from build123d import *

# Parameters (mm, degrees)
SKETCH1_W                        = 50.8
SKETCH1_H                        = 76.2
SKETCH1_R                        = 14.2875
BOSS_EXTRUDE1_DEPTH              = 8.89
F_10_CLEARANCE_HOLE1_D           = 5.1054
F_10_CLEARANCE_HOLE1_CSINK_D     = 6.3754
F_10_CLEARANCE_HOLE1_CSINK_ANGLE = 90


with BuildPart() as part:
    # Sketch1 → Boss-Extrude1 (new body)
    with BuildSketch(Plane.XY):
        with Locations((25.4, 38.1)):
            Rectangle(SKETCH1_W, SKETCH1_H)
        with Locations((25.4, 38.1)):
            Circle(SKETCH1_R, mode=Mode.SUBTRACT)
    extrude(amount=BOSS_EXTRUDE1_DEPTH)

    # #10 Clearance Hole1 (through all)
    with Locations(Plane.XY.offset(8.89)):
        with Locations((25.4, 66.675), (25.4, 9.525)):
            CounterSinkHole(F_10_CLEARANCE_HOLE1_D / 2, F_10_CLEARANCE_HOLE1_CSINK_D / 2, counter_sink_angle=F_10_CLEARANCE_HOLE1_CSINK_ANGLE)


solid = part.part
The model under review builds one solid part; all positions refer to its coordinate system, in mm. Give positions to 0.01 mm unless a question says otherwise; leave off trailing zeros. Order: outer loops, then holes, each group sorted by start corner. A loop starts at its lowest first (then second) coordinate and runs counter-clockwise, first axis right, second up. Notation, with made-up numbers: M 10.25,-4 L 68.25,-4 A24 cw 68.25,25 Z; hole C -5.5,52.5 d7. An arc over 180 degrees is marked long. Use one line per item in the form item = value. Start each with the question number.
Item 1: We need section A-A on x = 25.4. Give the boundary of the cut face in (y, z) (1 decimal).
Item 2: The part is to be moulded in two halves that separate along Y. For faces 1 (the flat face through (25, 76.2, 4)), 2 (the cylindrical face through (27.95, 9.64, 4.07)), 3 (the flat face through (50.8, 38, 4)), 4 (the cylindrical face through (14.06, 29.41, 4.38)), say which applies: pulls with the +Y half, pulls with the -Y half, needs draft (parallel to the pull), parting line crosses it, or undercut.
Item 3: We need section D-D on z = 7. Give the boundary of the cut face in (x, y) (1 decimal).
Item 4: We need section C-C on x = 35. Give the boundary of the cut face in (y, z), plus the area to 3 significant figures.
Item 5: To check wall thickness, follow line 1 along Y through (x, z) = (25.4, 5.5); line 2 along X through (y, z) = (66.5, 0.75); line 3 along Y through (x, z) = (34.5, 8.25). State the ranges of each line that lie inside material, in increasing order. Write a range as from..to.
Item 6: We need section B-B on y = 38.1. Give the boundary of the cut face in (x, z).
Completed:
q1.outline = M 0,0 L 7,0 L 7,8.3 L 6.3,8.9 L 0,8.9 Z; M 12.1,0 L 23.8,0 L 23.8,8.9 L 12.7,8.9 L 12.1,8.3 Z; M 52.4,0 L 64.1,0 L 64.1,8.3 L 63.5,8.9 L 52.4,8.9 Z; M 69.2,0 L 76.2,0 L 76.2,8.9 L 69.9,8.9 L 69.2,8.3 Z
q2.face_1 = pulls with the +Y half
q2.face_2 = undercut
q2.face_3 = needs draft
q2.face_4 = undercut
q3.outline = M 0,0 L 50.8,0 L 50.8,76.2 L 0,76.2 Z; hole C 25.4,38.1 d28.6; hole C 25.4,9.5 d5.1; hole C 25.4,66.7 d5.1
q4.outline = M 0,0 L 27.52,0 L 27.52,8.89 L 0,8.89 Z; M 48.68,0 L 76.2,0 L 76.2,8.89 L 48.68,8.89 Z
q4.area = 489 mm²
q5.line_1 = 0..6.97, 12.08..23.81, 52.39..64.12, 69.23..76.2
q5.line_2 = 0..22.85, 27.95..50.8
q5.line_3 = 0..27.09, 49.11..76.2
q6.outline = M 0,0 L 11.11,0 L 11.11,8.89 L 0,8.89 Z; M 39.69,0 L 50.8,0 L 50.8,8.89 L 39.69,8.89 Z
